from build123d import *

# Parameters (mm, degrees)
SKETCH1_W           = 12.3
SKETCH1_H           = 32.3
BOSS_EXTRUDE1_DEPTH = 5
SKETCH3_R           = 1
CUT_EXTRUDE1_DEPTH  = 285.989327178
SKETCH4_R           = 1
CUT_EXTRUDE2_DEPTH  = 249.777773307


with BuildPart() as part:
    # Sketch1 → Boss-Extrude1 (new body)
    with BuildSketch(Plane.XY.offset(6)):
        with Locations((-240.276643226, 268.361206467)):
            Rectangle(SKETCH1_W, SKETCH1_H)
    extrude(amount=BOSS_EXTRUDE1_DEPTH)

    # Sketch3 → Cut-Extrude1 (cut, through all)
    with BuildSketch(Plane.ZY.offset(246.426643226)):
        with Locations((8.542189851, 274.911206467)):
            Circle(SKETCH3_R)
        with Locations((8.542189851, 266.611206467)):
            Circle(SKETCH3_R)
    extrude(amount=-CUT_EXTRUDE1_DEPTH, mode=Mode.SUBTRACT)

    # Sketch4 → Cut-Extrude2 (cut, through all)
    with BuildSketch(Plane(origin=(0, 252.211206467, 0), x_dir=(-1, 0, 0), z_dir=(0, -1, 0))):
        with Locations(Location((244.126643226, -8.5, 0), (0, 0, 90))):
            Circle(SKETCH4_R)
        with Locations(Location((236.426643226, -8.5, 0), (0, 0, 90))):
            Circle(SKETCH4_R)
    extrude(amount=-CUT_EXTRUDE2_DEPTH, mode=Mode.SUBTRACT)


solid = part.part
Part model, mm, in its own coordinate system. Give positions to 0.01 mm unless a question says otherwise; leave off trailing zeros. Write each loop counter-clockwise with the first axis right and the second up, starting at its lowest first coordinate (ties: lowest second). Pieces come first, ordered by that corner, then holes.
1) Cut at D-D on x = -235.75. Write the cut outline in (y, z), then the cut area to 3 significant figures.
Resolved:
outline: (252.21, 6) - (284.51, 6) - (284.51, 7.76) - (275.54, 7.76) arc R1 cw to (274.28, 7.76) - (267.24, 7.76) arc R1 cw to (265.98, 7.76) - (252.21, 7.76) - close; (252.21, 9.24) - (265.89, 9.24) arc R1 cw to (267.33, 9.24) - (274.19, 9.24) arc R1 cw to (275.63, 9.24) - (284.51, 9.24) - (284.51, 11) - (252.21, 11) - close
area: 113 mm2
2) Cut at C-C on y = 262.5. Write the cut outline in (x, z).
Resolved:
outline: (-246.43, 6) - (-234.13, 6) - (-234.13, 11) - (-246.43, 11) - close; hole circle Ø2 at (-244.13, 8.5); hole circle Ø2 at (-236.43, 8.5)
3) Probe L1, parallel to X at y = 277, z = 8.5; L2, parallel to X at y = 277, z = 9; L3, parallel to Y at x = -242, z = 9.35. List the from-to ranges inside material, lowest first.
Resolved:
L1: x = -246.43 to -245.13, -243.13 to -237.43, -235.43 to -234.13
L2: x = -246.43 to -244.99, -243.26 to -237.29, -235.56 to -234.13
L3: y = 252.21 to 266.02, 267.2 to 274.32, 275.5 to 284.51
4) Cut at B-B on x = -242.25. Write the cut outline in (y, z), then the cut area to 3 significant figures.
Resolved:
outline: (252.21, 6) - (284.51, 6) - (284.51, 11) - (252.21, 11) - close; hole circle Ø2 at (266.61, 8.54); hole circle Ø2 at (274.91, 8.54)
area: 155 mm2
5) Cut at A-A on x = -237. Write the cut outline in (y, z).
Resolved:
outline: (252.21, 6) - (284.51, 6) - (284.51, 7.68) - (275.42, 7.68) arc R1 cw to (274.4, 7.68) - (267.12, 7.68) arc R1 cw to (266.1, 7.68) - (252.21, 7.68) - close; (252.21, 9.32) - (265.98, 9.32) arc R1 cw to (267.24, 9.32) - (274.28, 9.32) arc R1 cw to (275.54, 9.32) - (284.51, 9.32) - (284.51, 11) - (252.21, 11) - close
6) Two-plate mould, pull along Z, no slides. Class faces 1 (the face through (-240, 269, 11)), 2 (the face through (-244.51, 268.135, 7.576)), 3 (the face through (-240, 252.211, 8)), 4 (the face through (-240.4, 266.9, 9.5)): released by +Z, released by -Z, zero draft, split by the parting line, or undercut.
Resolved:
face 1: released by +Z
face 2: undercut
face 3: zero draft
face 4: undercut
